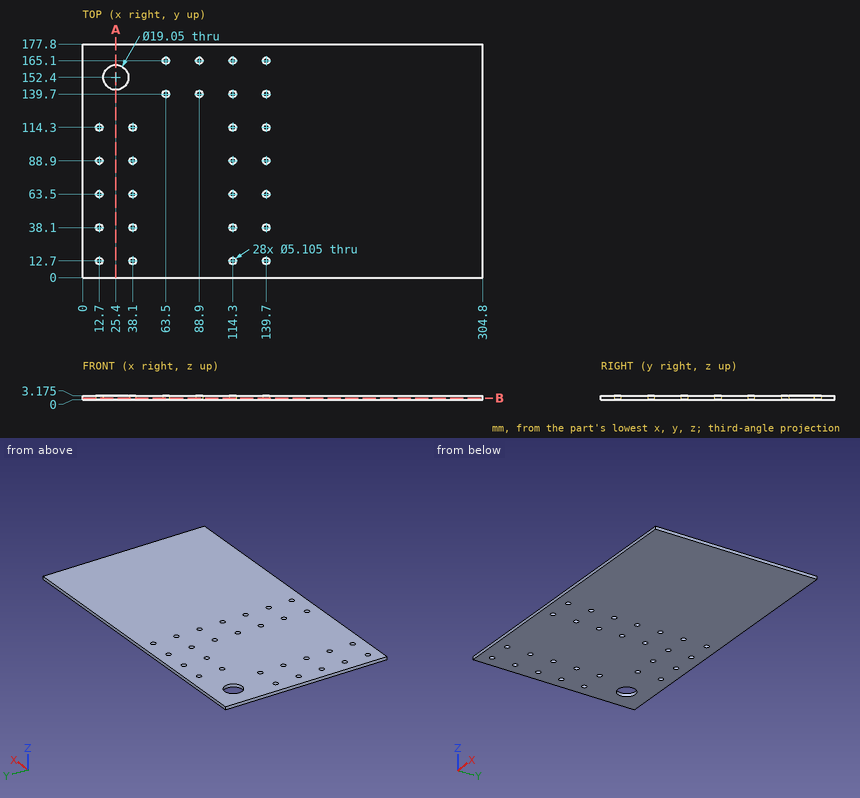
Part print with two shaded views. Sizes in mm from the minimum x, y, z corner. Give positions to 0.01 mm unless a question says otherwise; leave off trailing zeros. Loops run counter-clockwise (first coordinate to the right, second up) from the corner with the lowest first, then second, coordinate; pieces in that order, holes last. Notation, with made-up numbers: (64.5, 75.25) -> (118.5, 75.25) arc R22 cw to (118.5, 111.25) -> close; hole circle Ø8 at (-10, 63.5). An arc over 180 degrees is marked (long way). One line per question, with ' | ' between items.
Q1. Cut at A-A, the plane x = 25.4. Write the cut outline in (y, z) (1 decimal), plus the area to 3 significant figures.
Filled sheet:
outline: (0, 0) -> (142.9, 0) -> (142.9, 3.2) -> (0, 3.2) -> close; (161.9, 0) -> (177.8, 0) -> (177.8, 3.2) -> (161.9, 3.2) -> close | area: 504 mm²
Q2. Cut at B-B, the plane z = 1.2. Count the separate pieces of the cut face and the enclosed holes in it, plus the area to 3 significant figures.
Filled sheet:
separate pieces: 1 | enclosed holes: 29 | area: 53,300 mm²
Q3. Drop flat-ended pins along their axis: pin 1 (8 mm diameter, centred on x = 114.3, y = 165.1, fed in from -Z); pin 2 (3 mm diameter, centred on x = 38.1, y = 38.1, fed in from -Z). Give the stop position or say it passes through.
Filled sheet:
pin 1: stops at z = 0 | pin 2: passes through
Q4. Drill centre lines: line 1 along Y through (x, z) = (38.1, 2.1); line 2 along Y through (x, z) = (40, 1.15) (1 decimal); line 3 along X through (y, z) = (161, 1.55) (1 decimal). Where is each one in solid material? Low to high. Write a range as [from, to].
Filled sheet:
line 1: y = [0, 10.15], [15.25, 35.55], [40.65, 60.95], [66.05, 86.35], [91.45, 111.75], [116.85, 177.8] | line 2: y = [0, 11], [14.4, 36.4], [39.8, 61.8], [65.2, 87.2], [90.6, 112.6], [116, 177.8] | line 3: x = [0, 21.3], [29.5, 304.8]
